```python
from build123d import *

# Parameters (mm, degrees)
F0_W     = 4.6228
F0_H     = 4.6228
F0_W_2   = 292.1
F0_H_2   = 330.2
F1_DEPTH = 3.175


# Not quite as in the source:
# - a length typed as a fraction of an inch, garbled in the dataset ("3 / 203.2 mm" for 3/8 in), is restored


with BuildPart() as f1:
    # F0 (on Top) → F1 (new body)
    with BuildSketch(Plane.XY):
        Polygon((190.4998123646, 755.6496634722), (190.4998123646, 635.6350152016), (190.4998123646, 610.2350152016), (190.4998123646, 607.0600152016), (215.8998123646, 607.0600152016), (215.8998123646, 610.2350152016), (507.9998123646, 610.2350152016), (507.9998123646, 607.0600152016), (533.3998123646, 607.0600152016), (533.3998123646, 610.2350152016), (533.3998123646, 755.7291580558), (558.7998123646, 755.7291580558), (558.7998123646, 760.8061958763), (558.7998123646, 800.7350152016), (558.7998123646, 845.7408688016), (533.3998123646, 845.7408688016), (533.3998123646, 991.2350152016), (533.3998123646, 994.4100152016), (507.9998123646, 994.4100152016), (507.9998123646, 991.2350152016), (215.8998123646, 991.2350152016), (215.8998123646, 994.4100152016), (190.4998123646, 994.4100152016), (190.4998123646, 991.2350152016), (190.4998123646, 857.2496634722), align=None)
        with Locations((540.2533960062, 763.1175958763)):
            Rectangle(F0_W, F0_H, mode=Mode.SUBTRACT)
        with Locations((552.9533960062, 763.1175958763)):
            Rectangle(F0_W, F0_H, mode=Mode.SUBTRACT)
        with Locations((546.5928981277, 775.8096898529)):
            Rectangle(F0_W, F0_H, mode=Mode.SUBTRACT)
        with Locations((539.7752002493, 788.0271025263)):
            Rectangle(F0_W, F0_H, mode=Mode.SUBTRACT)
        with Locations((552.4752002493, 788.0271025263)):
            Rectangle(F0_W, F0_H, mode=Mode.SUBTRACT)
        with Locations((546.1356981277, 800.7350085497)):
            Rectangle(F0_W, F0_H, mode=Mode.SUBTRACT)
        with Locations((361.9498123646, 800.7350152016)):
            Rectangle(F0_W_2, F0_H_2, mode=Mode.SUBTRACT)
        with Locations((539.7752002493, 813.4271025263)):
            Rectangle(F0_W, F0_H, mode=Mode.SUBTRACT)
        with Locations((552.4752002493, 813.4271025263)):
            Rectangle(F0_W, F0_H, mode=Mode.SUBTRACT)
        with Locations((546.1356981277, 824.9666085497)):
            Rectangle(F0_W, F0_H, mode=Mode.SUBTRACT)
        with Locations((539.7752002493, 837.6587025263)):
            Rectangle(F0_W, F0_H, mode=Mode.SUBTRACT)
        with Locations((552.4752002493, 837.6587025263)):
            Rectangle(F0_W, F0_H, mode=Mode.SUBTRACT)
    extrude(amount=F1_DEPTH)


solid = f1.part
```
Can you work these out from the model? Positions are in its coordinate system, mm. Round coordinates to 2 decimals unless told otherwise and drop trailing zeros. Loops run counter-clockwise (first coordinate to the right, second up) from the corner with the lowest first, then second, coordinate; pieces in that order, holes last. Notation, with made-up numbers: M -23,58 L -8,58 A31 ccw -8,88 Z; hole C 42.5,8 d9. An arc over 180 degrees is marked long. Answer in a Markdown table with one row per item.
1. If we section it at B-B, the plane x = 228: Please give me the cut outline in (y, z) (3 decimals).
Established:
| item | result |
|---|---|
| outline | M 610.235,0 L 635.635,0 L 635.635,3.175 L 610.235,3.175 Z; M 965.835,0 L 991.235,0 L 991.235,3.175 L 965.835,3.175 Z |
2. If we section it at A-A, the plane y = 958: Please give me the cut outline in (x, z) (3 decimals).
Established:
| item | result |
|---|---|
| outline | M 190.5,0 L 215.9,0 L 215.9,3.175 L 190.5,3.175 Z; M 508,0 L 533.4,0 L 533.4,3.175 L 508,3.175 Z |
3. If we section it at C-C, the plane z = 1.2: Give the number of separate pieces and of enclosed holes in the cut face, plus the area to 3 significant figures.
Established:
| item | result |
|---|---|
| separate pieces | 1 |
| enclosed holes | 12 |
| area | 36,600 mm² |
4. Please list where these lines run through material, in increasing order: line 1 (Y direction, x = 375.5, z = 1.4); line 2 (X direction, y = 954, z = 3.05); line 3 (X direction, y = 809, z = 1.9). Write a range as from..to.
Established:
| item | result |
|---|---|
| line 1 | 610.24..635.64, 965.84..991.24 |
| line 2 | 190.5..215.9, 508..533.4 |
| line 3 | 190.5..215.9, 508..558.8 |
5. I'm going to push flat-ended pins straight in: pin 1 Ø1.6 at (x, z) = (540.5, 1.5) entering from -Y; pin 2 Ø1.6 at (x, z) = (540.5, 1.5) entering from +Y; pin 3 Ø1.5 at (x, z) = (502, 2) entering from -Y (3 decimals). Where does each tip first touch, or does it pass through?
Established:
| item | result |
|---|---|
| pin 1 | y = 755.73 |
| pin 2 | y = 845.74 |
| pin 3 | y = 610.235 |
